Read the model definition and answer for the solid it produces. Units are mm, in the model's axes. Face numbers are marked on the shaded views. A direction names the side the tool comes from. Coordinates: 2 decimals unless noted, no trailing zeros. Order: outer loops, then holes, each group sorted by start corner. A loop starts at its lowest first (then second) coordinate and runs counter-clockwise, first axis right, second up. Notation, with made-up numbers: (19.5, -40) -> (40.5, -40) arc R23 cw to (40.5, -6) -> close; hole circle Ø2 at (-23, 76). An arc over 180 degrees is marked (long way). Use CSV: the item, a comma, the result in double quotes.
```python
from build123d import *

# Parameters (mm, degrees)
SKETCH1_R           = 3.5
BOSS_EXTRUDE1_DEPTH = 11.5
FILLET1_R           = 3.5
SKETCH3_W           = 8
SKETCH3_H           = 8
BOSS_EXTRUDE2_DEPTH = 1.2
CHAMFER1_SIZE       = 0.5
CHAMFER2_SIZE       = 0.5


with BuildPart() as part:
    # Sketch1 → Boss-Extrude1 (new body)
    with BuildSketch(Plane.XY):
        Circle(SKETCH1_R)
    extrude(amount=BOSS_EXTRUDE1_DEPTH)

    # Fillet1
    fillet1_edges = [part.edges().sort_by_distance(p)[0] for p in [
        (-3.5, 0, 11.5),
    ]]
    fillet(fillet1_edges, radius=FILLET1_R)

    # Sketch3 → Boss-Extrude2 (add)
    with BuildSketch(Plane(origin=(0, 0, 2), x_dir=(-1, 0, 0), z_dir=(0, 0, -1))):
        Rectangle(SKETCH3_W, SKETCH3_H)
    extrude(amount=-BOSS_EXTRUDE2_DEPTH)

    # Chamfer1
    chamfer1_edges = [part.edges().sort_by_distance(p)[0] for p in [
        (-3.5, 0, 0),
    ]]
    chamfer(chamfer1_edges, length=CHAMFER1_SIZE)

    # Chamfer2
    chamfer2_edges = [part.edges().sort_by_distance(p)[0] for p in [
        (4, 0, 2),
        (0, -4, 2),
        (-4, 0, 2),
        (0, 4, 2),
    ]]
    chamfer(chamfer2_edges, length=CHAMFER2_SIZE - 0.0001)  # a hair under: the kernel refuses the full size


solid = part.part
```
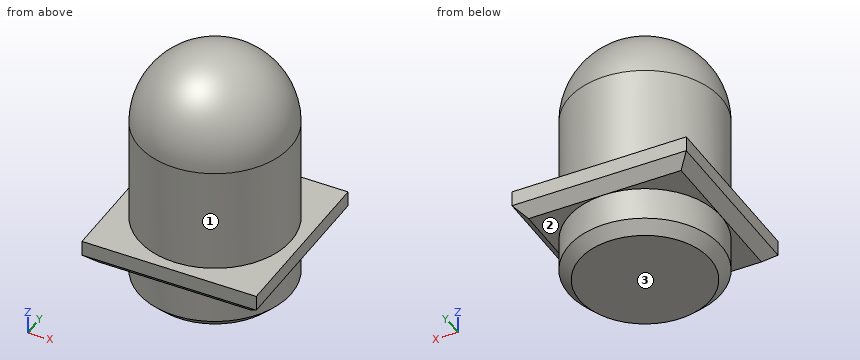
Item 1: Straight lines are drawn through the part: line 1 along Y through (x, z) = (0, 7.5); line 2 along Z through (x, y) = (3.25, 2.25); line 3 along Y through (x, z) = (2.5, 1.5). For each, find the intervals that lie inside material, in ascending order.
Return value:
line 1,"y = -3.5 to 3.5"
line 2,"z = 2 to 3.2"
line 3,"y = -2.45 to 2.45"
Item 2: Each of these flat-tipped pins is pushed along its axis until it touches: P1, Ø1, axis at y = 2, z = 5, coming from the -X side; P2, Ø2, axis at x = -3, y = -2, coming from the +Z side; P3, Ø1.5, axis at x = -2.5, y = -0.5, coming from the +Z side. Where does it stop, or does it pass through?
Return value:
P1,"stops at x = -3.16"
P2,"stops at z = 10.34"
P3,"stops at z = 11"
Item 3: A tool of negligible diameter and unlimited length cuts with its end or side. For the marked faces 1, 2 and 3, from which of +Z, -Z, +X, -X, +Y, -Y can it reach the whole face along a straight path? Write none if from no direction.
Return value:
face 1,"+Z"
face 2,"-Z"
face 3,"-Z, +X, -X, +Y, -Y"
Item 4: Find section B-B, the plane z = 9. Give the vertices of the cut face in (x, y).
Return value:
outline,"circle Ø6.71 at (0, 0)"
Item 5: Find section A-A, the plane z = 5.25. Give the vertices of the cut face in (x, y).
Return value:
outline,"circle Ø7 at (0, 0)"
